Geometry check sheet. Reference: the model listing, model coordinates, mm. Face numbers are marked on the shaded views. A direction names the side the tool comes from. Coordinates: 2 decimals unless noted, no trailing zeros. Loops run counter-clockwise (first coordinate to the right, second up) from the corner with the lowest first, then second, coordinate; pieces in that order, holes last.
from build123d import *

# Parameters (mm, degrees)
F1_DEPTH = 60
F2_R     = 5
F3_R     = 25
F4_DEPTH = 25


with BuildPart() as f1:
    # F0 (on Front) → F1 (new body)
    with BuildSketch(Plane.XZ):
        with BuildLine():
            Line((9.088148, 68.306795), (-40.911852, 68.306795))
            ThreePointArc((-40.911852, 68.306795), (-58.589521, 60.984465), (-65.911852, 43.306795))
            Line((-65.911852, 43.306795), (-65.911852, -6.693205))
            ThreePointArc((-65.911852, -6.693205), (-58.589521, -24.370874), (-40.911852, -31.693205))
            Line((-40.911852, -31.693205), (9.088148, -31.693205))
            ThreePointArc((9.088148, -31.693205), (26.765818, -24.370874), (34.088148, -6.693205))
            Line((34.088148, -6.693205), (34.088148, 43.306795))
            ThreePointArc((34.088148, 43.306795), (26.765818, 60.984465), (9.088148, 68.306795))
        make_face()
    extrude(amount=F1_DEPTH)

    # F2
    f2_edges = [f1.edges().sort_by_distance(p)[0] for p in [
        (-15.911852, -60, 68.306795),
        (-58.589521, -60, 60.984465),
        (-65.911852, -60, 18.306795),
        (-58.589521, -60, -24.370874),
        (-15.911852, -60, -31.693205),
        (26.765818, -60, -24.370874),
        (34.088148, -60, 18.306795),
        (26.765818, -60, 60.984465),
        (-15.911852, 0, 68.306795),
        (-58.589521, 0, 60.984465),
        (-65.911852, 0, 18.306795),
        (-58.589521, 0, -24.370874),
        (-15.911852, 0, -31.693205),
        (26.765818, 0, -24.370874),
        (34.088148, 0, 18.306795),
        (26.765818, 0, 60.984465),
    ]]
    fillet(f2_edges, radius=F2_R)

    # F3 (on face) → F4 (cut)
    with BuildSketch(Plane.XZ.offset(60)):
        with Locations((-15.923823, 19.471144)):
            Circle(F3_R)
    extrude(amount=-F4_DEPTH, mode=Mode.SUBTRACT)


solid = f1.part
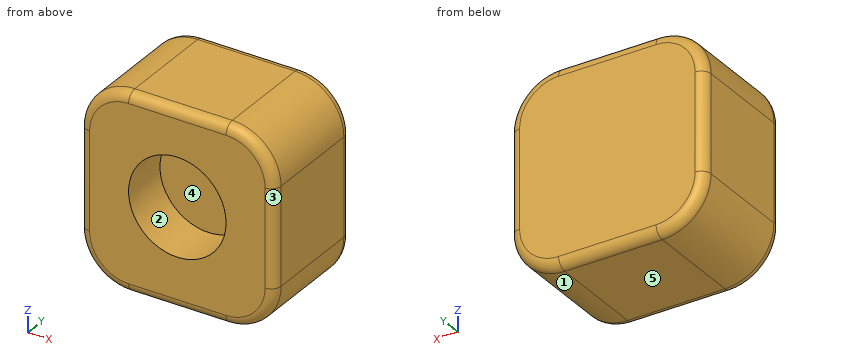
(1) Sectioned sample at C-C on y = -32.5. Record the cut outline in (x, z), and give its area (3 significant figures).
Findings:
outline: (-65.91, -6.69) arc R25 ccw to (-40.91, -31.69) - (9.09, -31.69) arc R25 ccw to (34.09, -6.69) - (34.09, 43.31) arc R25 ccw to (9.09, 68.31) - (-40.91, 68.31) arc R25 ccw to (-65.91, 43.31) - close
area: 9,460 mm2
(2) Gauge pin test, flat ends, axial feed: pin 1 Ø2 at (y, z) = (-47, 55) entering from -X; pin 2 Ø3 at (x, y) = (16.5, -18) entering from -Z; pin 3 Ø2 at (x, y) = (-51, -28) entering from -Z. Record the tip position at first contact, or that the pin passes through.
Findings:
pin 1: stops at x = -63.51
pin 2: stops at z = -30.98
pin 3: stops at z = -29.98
(3) Sectioned sample at D-D on x = -31. Record the cut outline in (y, z), and give its area (3 significant figures).
Findings:
outline: (-60, -26.69) arc R5 ccw to (-55, -31.69) - (-5, -31.69) arc R5 ccw to (0, -26.69) - (0, 63.31) arc R5 ccw to (-5, 68.31) - (-55, 68.31) arc R5 ccw to (-60, 63.31) - (-60, 39.41) - (-35, 39.41) - (-35, -0.47) - (-60, -0.47) - close
area: 4,980 mm2
(4) Scan lines: L1, parallel to Z at x = -42, y = -49; L2, parallel to X at y = -40, z = 39.5; L3, parallel to Z at x = -32.5, y = -41. Record each from-to range of solid material in increasing order.
Findings:
L1: z = -31.67 to 68.28
L2: x = -65.91 to -30.89, -0.96 to 34.09
L3: z = -31.69 to 0.76, 38.19 to 68.31
(5) Sectioned sample at B-B on z = 39.5. Record the cut outline in (x, y), and give its area (3 significant figures).
Findings:
outline: (-65.91, -55) arc R5 ccw to (-60.91, -60) - (-30.89, -60) - (-30.89, -35) - (-0.96, -35) - (-0.96, -60) - (29.09, -60) arc R5 ccw to (34.09, -55) - (34.09, -5) arc R5 ccw to (29.09, 0) - (-60.91, 0) arc R5 ccw to (-65.91, -5) - close
area: 5,230 mm2
(6) Access from +Z, -Z, +X, -X, +Y, -Y to the whole of each face (thin tool, end or side, straight path). Record for the marked faces 4 and 5.
Findings:
face 4: -Y
face 5: -Z, +X, -X, +Y, -Y
(7) Sectioned sample at A-A on y = -40.5. Record the cut outline in (x, z), and give its area (3 significant figures).
Findings:
outline: (-65.91, -6.69) arc R25 ccw to (-40.91, -31.69) - (9.09, -31.69) arc R25 ccw to (34.09, -6.69) - (34.09, 43.31) arc R25 ccw to (9.09, 68.31) - (-40.91, 68.31) arc R25 ccw to (-65.91, 43.31) - close; hole circle Ø50 at (-15.92, 19.47)
area: 7,500 mm2
(8) Draft check along Z on the marked faces 1, 2 and 3. Enter one of: +Z half, -Z half, draft (parallel to the pull), parting line (faces both ways), or undercut.
Findings:
face 1: -Z half
face 2: undercut
face 3: draft
